Source: CAD feature listing. Evaluate the final solid. Frame: model axes, mm. A direction names the side the tool comes from. Round coordinates to 2 decimals unless told otherwise and drop trailing zeros. Order: outer loops, then holes, each group sorted by start corner. A loop starts at its lowest first (then second) coordinate and runs counter-clockwise, first axis right, second up. Notation, with made-up numbers: (-9, 68) - (2, 68) arc R11 cw to (2, 72) - close; hole circle Ø3 at (78, 23). An arc over 180 degrees is marked (long way). Return JSON: item names as keys, results as strings. Group by question number.
1) Section B-B, the plane z = 13.25. Return loops of the section in (x, y), plus the area to 3 significant figures.
2) Section C-C, the plane y = 50.5. Return loops of the section in (x, z), plus the area to 3 significant figures.
3) Contact query for flat-ended pins moving along their axis: P1, Ø1.5, axis at x = 40.5, y = -55.5, coming from the -Z side; P2, Ø8, axis at x = 88.86, y = 0, coming from the -Z side; P3, Ø16, axis at x = -89.71, y = -38.96, coming from the -Z side; P4, Ø20.5, axis at x = 94.01, y = 44.89, coming from the -Z side. Output: stop coordinate, or through.
4) Access query for faces 4 (the cylindrical face through (-83.27, -44.88, 20.77)), 5 (the flat face through (85, 48, 16)). Directions: +Z, -Z, +X, -X, +Y, -Y. A direction counts if a zero-diameter tool reaches every point of the face in a straight line with its end or side. Return the directions, or none.
5) Mould query, pull axis Y, two halves, no side actions, for faces 1 (the cylindrical face through (1.707, -74.751, 1.528)), 2 (the cylindrical face through (-88.96, 14.56, 2.46)), 3 (the cylindrical face through (-125.551, 74.672, 12.807)). Classes: pulls with the +Y half, pulls with the -Y half, needs draft (parallel to the pull), parting line crosses it, or undercut.
6) Ray query, line 1 (X direction, y = -38.5, z = 6.5); line 2 (X direction, y = -24.5, z = 14); line 3 (Y direction, x = 68, z = 20.75). Return the intervals inside material, ascending. Write a range as from..to.
7) Section A-A, the plane y = 0. Return loops of the section in (x, z), plus the area to 3 significant figures.
```python
from build123d import *

# Parameters (mm, degrees)
F0_W           = 254
F0_H           = 152.4
F1_DEPTH       = 25.4
F2_R           = 5.08
F4_D           = 17.5
F4_CBORE_D     = 25.5
F4_CBORE_DEPTH = 16
F6_D           = 5.5
F6_CBORE_D     = 9.75
F6_CBORE_DEPTH = 5


with BuildPart() as f1:
    # F0 (on Top) → F1 (new body)
    with BuildSketch(Plane.XY):
        Rectangle(F0_W, F0_H)
    extrude(amount=F1_DEPTH)

    # F2
    f2_edges = [f1.edges().sort_by_distance(p)[0] for p in [
        (127, 0, 25.4),
        (0, 76.2, 25.4),
        (-127, 0, 25.4),
        (0, -76.2, 25.4),
        (127, 76.2, 12.7),
        (-127, 76.2, 12.7),
        (0, 76.2, 0),
        (127, -76.2, 12.7),
        (127, 0, 0),
        (-127, -76.2, 12.7),
        (0, -76.2, 0),
        (-127, 0, 0),
    ]]
    fillet(f2_edges, radius=F2_R)

    # F4 (through all)
    with Locations(Plane(origin=(0, 0, 0), x_dir=(1, 0, 0), z_dir=(0, 0, -1))):
        with Locations((107.5116768479, 28.6860521883), (94.0102785826, -44.8912791908), (-89.7149518132, 38.9632694423)):
            CounterBoreHole(F4_D / 2, F4_CBORE_D / 2, F4_CBORE_DEPTH)

    # F6 (through all)
    with Locations(Plane(origin=(0, 0, 0), x_dir=(1, 0, 0), z_dir=(0, 0, -1))):
        with Locations((-93.461304903, -12.6921338961), (88.8565033674, 0), (86.5757465363, 51.5028946102)):
            CounterBoreHole(F6_D / 2, F6_CBORE_D / 2, F6_CBORE_DEPTH)


solid = f1.part
```
Geometry check:
{
 "1": {"outline": "(-127, -71.12) arc R5.08 ccw to (-121.92, -76.2) - (121.92, -76.2) arc R5.08 ccw to (127, -71.12) - (127, 71.12) arc R5.08 ccw to (121.92, 76.2) - (-121.92, 76.2) arc R5.08 ccw to (-127, 71.12) - close; hole circle Ø25.5 at (-89.71, -38.96); hole circle Ø5.5 at (-93.46, 12.69); hole circle Ø25.5 at (94.01, 44.89); hole circle Ø5.5 at (86.58, -51.5); hole circle Ø5.5 at (88.86, 0); hole circle Ø25.5 at (107.51, -28.69)", "area": "37,100 mm2"},
 "2": {"outline": "(-127, 5.08) arc R5.08 ccw to (-121.92, 0) - (82.56, 0) - (82.56, 16) - (87.29, 16) - (87.29, 25.4) - (-121.92, 25.4) arc R5.08 ccw to (-127, 20.32) - close; (100.73, 16) - (105.46, 16) - (105.46, 0) - (121.92, 0) arc R5.08 ccw to (127, 5.08) - (127, 20.32) arc R5.08 ccw to (121.92, 25.4) - (100.73, 25.4) - close", "area": "5,940 mm2"},
 "3": {"P1": "z = 0", "P2": "z = 5", "P3": "through", "P4": "z = 16"},
 "4": {"face 4": "+Z, -Z", "face 5": "-Z"},
 "5": {"face 1": "pulls with the -Y half", "face 2": "undercut", "face 3": "pulls with the +Y half"},
 "6": {"line 1": "-127..-102.46, -76.97..99.37, 115.65..127", "line 2": "-127..95.47, 119.55..127", "line 3": "-76.18..76.18"},
 "7": {"outline": "(-127, 5.08) arc R5.08 ccw to (-121.92, 0) - (83.98, 0) - (83.98, 5) - (86.11, 5) - (86.11, 25.4) - (-121.92, 25.4) arc R5.08 ccw to (-127, 20.32) - close; (91.61, 5) - (93.73, 5) - (93.73, 0) - (121.92, 0) arc R5.08 ccw to (127, 5.08) - (127, 20.32) arc R5.08 ccw to (121.92, 25.4) - (91.61, 25.4) - close", "area": "6,270 mm2"}
}
